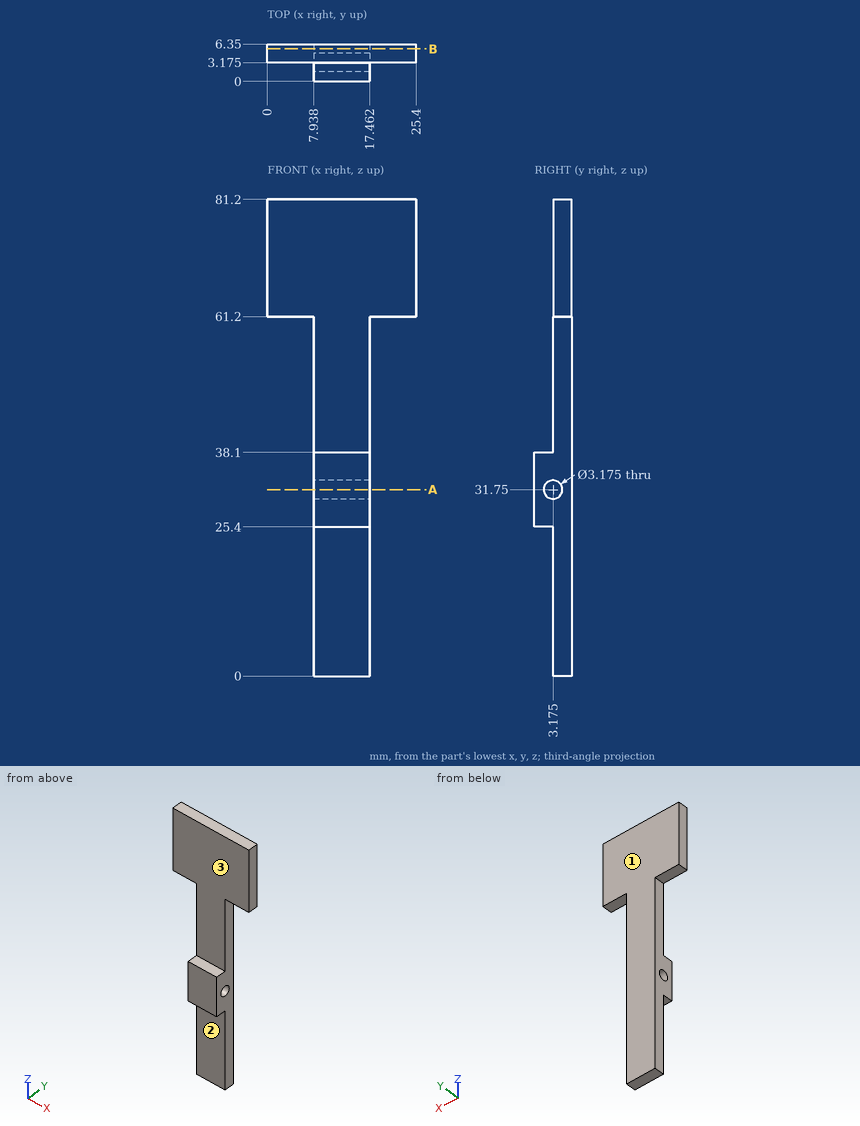
Job drawing, mm, ordinate dimensions from the low corner. One solid piece. A direction names the side the tool comes from. Give positions to 0.01 mm unless a question says otherwise; leave off trailing zeros. Loops run counter-clockwise (first coordinate to the right, second up) from the corner with the lowest first, then second, coordinate; pieces in that order, holes last. Notation, with made-up numbers: (73.25, 74.25) - (91.25, 74.25) arc R27 ccw to (91.25, 112.25) - close; hole circle Ø1 at (-4, 27). An arc over 180 degrees is marked (long way). Use one line per item in the form item = value.
(1) Drop flat-ended pins along their axis: P1, Ø1.6, axis at x = 4.5, y = 5, coming from the -Z side; P2, Ø6, axis at x = 15.5, z = 14, coming from the -Y side (1 decimal); P3, Ø1, axis at x = 11.5, y = 1, coming from the +Z side; P4, Ø3, axis at y = 3.175, z = 31.75, coming from the -X side. Give the stop position or say it passes through.
Determined:
P1 = 61.2
P2 = 3.2
P3 = 38.1
P4 = through
(2) Cut at B-B (y = 5.5). Give the cut face in (x, z).
Determined:
outline = (0, 61.2) - (7.94, 61.2) - (7.94, 0) - (17.46, 0) - (17.46, 61.2) - (25.4, 61.2) - (25.4, 81.2) - (0, 81.2) - close
(3) Cut at A-A (z = 31.75). Give the cut face in (x, y).
Determined:
outline = (7.94, 0) - (17.46, 0) - (17.46, 1.59) - (7.94, 1.59) - close; (7.94, 4.76) - (17.46, 4.76) - (17.46, 6.35) - (7.94, 6.35) - close
(4) 3-axis set-ups, long thin cutter, end or side, ignore diameter. For the marked faces 1, 2 and 3: which of +Z, -Z, +X, -X, +Y, -Y reach the whole face in a straight line?
Determined:
face_1 = +Z, -Z, +X, -X, +Y
face_2 = -Z, +X, -X, -Y
face_3 = +Z, +X, -X, -Y
(5) Drill centre lines: L1, parallel to Y at x = 14.25, z = 31.75; L2, parallel to X at y = 4.5, z = 30; L3, parallel to Z at x = 4.75, y = 4.75. Where is each one in solid material? Low to high.
Determined:
L1 = 0 to 1.59, 4.76 to 6.35
L2 = 7.94 to 17.46
L3 = 61.2 to 81.2
